Autodesk Inventor part; units mm, degrees
ref_plane "YZ Plane" through (0, 0, 0) normal (1, 0, 0) x (0, 1, 0)
ref_plane "XZ Plane" through (0, 0, 0) normal (0, 1, 0) x (-1, 0, 0)
ref_plane "XY Plane" through (0, 0, 0) normal (0, 0, 1) x (1, 0, 0)
sketch "Sketch1" plane through (0, 0, 0) normal (0, 1, 0) x (-1, 0, 0)
  line L0 (38.1, 76.2) -> (-63.5, 76.2)
  line L1 (-63.5, 76.2) -> (-63.5, -76.2)
  line L2 (-63.5, -76.2) -> (38.1, -76.2)
  line L3 (38.1, -76.2) -> (38.1, 76.2)
  circle A0 centre (-50.8, -31.75) radius 3.9751
  circle A1 centre (12.7, 69.85) radius 3.175
  circle A2 centre (12.7, -69.85) radius 3.175
  point P0 (0, 0)
  point P1 (38.1, 0)
  dimension "d0" = 152.4
  dimension "d1" = 101.6
  dimension "d2" = 38.1
  dimension "d6" = 7.9502
  dimension "d7" = 6.35
  dimension "d8" = 6.35
  dimension "d9" = 25.4
  dimension "d10" = 6.35
  dimension "d11" = 6.35
  dimension "d12" = 25.4
  dimension "d14" = 107.95
  dimension "d15" = 88.9
extrude "Extrusion1" add sketch "Sketch1" along normal blind 25.4
properties part number "Top Plate for Side to Side motion"
Could you check a few things on this model? Use its own coordinates, in mm. Give positions to 0.01 mm unless a question says otherwise; leave off trailing zeros. Order: outer loops, then holes, each group sorted by start corner. A loop starts at its lowest first (then second) coordinate and runs counter-clockwise, first axis right, second up.
1. Will this pin go through, and if not, where does the flat tip stop? P1, Ø4, axis at x = 51.5, z = 11.5, coming from the -Y side.
2. Suppose I cut it at A-A (x = -12.7). List the corners of the cut face in (y, z) for me (3 decimals).
3. Suppose I cut it at C-C (z = -69.85). List the corners of the cut face in (x, y) for me (3 decimals), plus the area to 3 significant figures.
4. We'd pull the mould along X, two halves only. Please class faces 1 (the flat face through (13, 13, -76.2)), 2 (the flat face through (-38.1, 13, -1)), 3 (the cylindrical face through (51.32, 12.52, -35.69)): pulls with the +X half, pulls with the -X half, needs draft (parallel to the pull), parting line crosses it, or undercut.
5. Suppose I cut it at B-B (z = -31.75). List the corners of the cut face in (x, y) for me.
6. I need wall thicknesses on L1, parallel to Z at x = 50.8, y = 18.75; L2, parallel to Z at x = -12.7, y = 14.25 (3 decimals); L3, parallel to X at y = 4, z = 67. Which ranges of each line are inside material? Lowest first, please.
Solved:
1. P1: stops at y = 0
2. outline: (0, -76.2) - (25.4, -76.2) - (25.4, -73.025) - (0, -73.025) - close; (0, -66.675) - (25.4, -66.675) - (25.4, 66.675) - (0, 66.675) - close; (0, 73.025) - (25.4, 73.025) - (25.4, 76.2) - (0, 76.2) - close
3. outline: (-38.1, 0) - (-15.875, 0) - (-15.875, 25.4) - (-38.1, 25.4) - close; (-9.525, 0) - (63.5, 0) - (63.5, 25.4) - (-9.525, 25.4) - close
3. area: 2,420 mm2
4. face 1: needs draft
4. face 2: pulls with the -X half
4. face 3: undercut
5. outline: (-38.1, 0) - (46.82, 0) - (46.82, 25.4) - (-38.1, 25.4) - close; (54.78, 0) - (63.5, 0) - (63.5, 25.4) - (54.78, 25.4) - close
6. L1: z = -76.2 to -35.73, -27.77 to 76.2
6. L2: z = -76.2 to -73.025, -66.675 to 66.675, 73.025 to 76.2
6. L3: x = -38.1 to -14.1, -11.3 to 63.5
